```python
from build123d import *

# Parameters (mm, degrees)
SKETCH1_W           = 94
SKETCH1_H           = 130
BOSS_EXTRUDE1_DEPTH = 9.5
SKETCH2_W           = 90.5
SKETCH2_H           = 126.5
CUT_EXTRUDE1_DEPTH  = 2.5
SKETCH3_W           = 72
SKETCH3_H           = 24
CUT_EXTRUDE2_DEPTH  = 8
SKETCH4_W           = 70
SKETCH4_H           = 78
CUT_EXTRUDE3_DEPTH  = 2
SKETCH5_W           = 23
SKETCH5_H           = 3.5
CUT_EXTRUDE4_DEPTH  = 8.5
SKETCH6_W           = 6
SKETCH6_H           = 18
CUT_EXTRUDE5_DEPTH  = 3.5
SKETCH7_W           = 43
SKETCH7_H           = 7.5
CUT_EXTRUDE6_DEPTH  = 3
FILLET1_R           = 2
BOSS_EXTRUDE3_DEPTH = 2


with BuildPart() as part:
    # Sketch1 → Boss-Extrude1 (new body)
    with BuildSketch(Plane(origin=(0, 7, 0), x_dir=(1, 0, 0), z_dir=(0, 1, 0))):
        with Locations((47, 65)):
            Rectangle(SKETCH1_W, SKETCH1_H)
    extrude(amount=-BOSS_EXTRUDE1_DEPTH)

    # Sketch2 → Cut-Extrude1 (cut)
    with BuildSketch(Plane.XZ.offset(2.5)):
        with Locations((47, -65)):
            Rectangle(SKETCH2_W, SKETCH2_H)
    extrude(amount=-CUT_EXTRUDE1_DEPTH, mode=Mode.SUBTRACT)

    # Sketch3 → Cut-Extrude2 (cut, through all)
    with BuildSketch(Plane.XZ):
        with Locations((47, -100)):
            Rectangle(SKETCH3_W, SKETCH3_H)
    extrude(amount=-CUT_EXTRUDE2_DEPTH, mode=Mode.SUBTRACT)

    # Sketch4 → Cut-Extrude3 (cut)
    with BuildSketch(Plane(origin=(0, 7, 0), x_dir=(-1, 0, 0), z_dir=(0, 1, 0))):
        with Locations((-42, -44)):
            Rectangle(SKETCH4_W, SKETCH4_H)
    extrude(amount=-CUT_EXTRUDE3_DEPTH, mode=Mode.SUBTRACT)

    # Sketch5 → Cut-Extrude4 (cut, through all)
    with BuildSketch(Plane(origin=(0, 5, 0), x_dir=(-1, 0, 0), z_dir=(0, 1, 0))):
        with Locations((-42, -9.25)):
            Rectangle(SKETCH5_W, SKETCH5_H)
    extrude(amount=-CUT_EXTRUDE4_DEPTH, mode=Mode.SUBTRACT)

    # Sketch6 → Cut-Extrude5 (cut)
    with BuildSketch(Plane.XZ):
        with Locations((86, -100)):
            Rectangle(SKETCH6_W, SKETCH6_H)
    extrude(amount=-CUT_EXTRUDE5_DEPTH, mode=Mode.SUBTRACT)

    # Sketch7 → Cut-Extrude6 (cut)
    with BuildSketch(Plane.XZ):
        with Locations((33.5, -115.75)):
            Rectangle(SKETCH7_W, SKETCH7_H)
    extrude(amount=-CUT_EXTRUDE6_DEPTH, mode=Mode.SUBTRACT)

    # Fillet1
    fillet1_edges = [part.edges().sort_by_distance(p)[0] for p in [
        (94, 7, -65),
        (47, 7, 0),
        (0, 7, -65),
        (47, 7, -130),
        (94, 2.25, -130),
        (94, 2.25, 0),
        (0, 2.25, 0),
        (0, 2.25, -130),
    ]]
    fillet(fillet1_edges, radius=FILLET1_R)

    # Sketch10 → Boss-Extrude3 (add)
    with BuildSketch(Plane(origin=(0, 7, 0), x_dir=(1, 0, 0), z_dir=(0, 1, 0))):
        Polygon((26.5, 123), (24.5, 125), (20.5, 125), (18.5, 123), (18.5, 117), (20.5, 115), (24.5, 115), (25, 115.309128344), (25, 115), (26.5, 115), (26.5, 120), (22.5, 120), (22.5, 118.5), (25, 118.5), (25, 117.072659745), (24.07375083, 116.5), (21.121320344, 116.5), (20, 117.621320344), (20, 122.367836714), (21.110870681, 123.5), (23.878679656, 123.5), (25, 122.378679656), (26.5, 122.378679656), align=None)
        Polygon((32.378679656, 119), (30.5, 119), (30.5, 115), (29, 115), (29, 125), (34.5, 125), (36, 123.5), (36, 120.5), (34.5, 119), (36, 117.5), (36, 115), (34.5, 115), (34.5, 116.878679656), align=None)
        Polygon((30.5, 123.496173662), (30.5, 120.5), (33.882505994, 120.5), (34.5, 121.117494006), (34.5, 122.878679656), (33.882505994, 123.496173662), align=None, mode=Mode.SUBTRACT)
        Polygon((43.5, 125), (45.5, 123.276052985), (45.5, 117.021376869), (43.5, 115), (40.272028005, 115), (38.5, 117.021376869), (38.5, 123.276052985), (40.272028005, 125), align=None)
        Polygon((42.942743976, 123.5), (44, 122.588673317), (44, 117.638031489), (42.874003649, 116.5), (40.951839055, 116.5), (40, 117.585775983), (40, 122.642614002), (40.881298547, 123.5), align=None, mode=Mode.SUBTRACT)
        Polygon((48, 117), (50, 115), (53, 115), (55, 117), (55, 125), (53.5, 125), (53.5, 123.5), (53.5, 117.621320344), (52.378679656, 116.5), (50.621320344, 116.5), (49.5, 117.621320344), (49.5, 123.5), (49.5, 125), (48, 125), align=None)
        Polygon((63, 119), (59, 119), (59, 115), (57.5, 115), (57.5, 125), (63, 125), (64.5, 123.5), (64.5, 120.5), align=None)
        Polygon((59, 123.5), (59, 120.5), (62.378679656, 120.5), (63, 121.121320344), (63, 122.878679656), (62.378679656, 123.5), align=None, mode=Mode.SUBTRACT)
    extrude(amount=BOSS_EXTRUDE3_DEPTH)


solid = part.part
```
Can you work these out from the model? Positions are in its coordinate system, mm. A direction names the side the tool comes from. Round coordinates to 2 decimals unless told otherwise and drop trailing zeros. Loops run counter-clockwise (first coordinate to the right, second up) from the corner with the lowest first, then second, coordinate; pieces in that order, holes last.
Item 1: Suppose I cut it at C-C, the plane x = 86.5. Write out the boundary of the cut face in (y, z).
Item 2: If we mould it in two halves opening along X, with no side actions, what happens to faces 6 (the flat face through (0, 1, -64)), 7 (the flat face through (30.5, 3, -9)), 8 (the flat face through (60, 9, -120)), 9 (the flat face through (61, 7, -122))? For each: +X half, -X half, draft (parallel to the pull), parting line (faces both ways), or undercut.
Item 3: Suppose I cut it at A-A, the plane z = -102.5. Write out the boundary of the cut face in (x, y), then the cut area to 3 significant figures.
Item 4: Suppose I cut it at B-B, the plane x = 69.5. Write out the boundary of the cut face in (y, z).
Item 5: Suppose I cut it at D-D, the plane z = -66. Write out the boundary of the cut face in (x, y), then the cut area to 3 significant figures.
Item 6: Will these pins go through, and if not, where does the flat tip stop? pin 1 Ø1.6 at (x, y) = (48.5, 8) entering from -Z; pin 2 Ø0.6 at (x, y) = (51.5, 7.5) entering from +Z; pin 3 Ø2 at (x, z) = (31, -63) entering from +Y.
Item 7: Which directions (+Z, -Z, +X, -X, +Y, -Y) give clear straight access to the entire face, cutting with the end or side of a thin tool? Please do faces 1 (the flat face through (44.4, 9, -120.1)), 2 (the flat face through (94, 1, -64)), 3 (the flat face through (86, 2, -109)), 4 (the flat face through (42, 3, -7.5)), 5 (the flat face through (42, 7, -120)).
Item 8: Please list where these lines run through material, in increasing order: L1, parallel to Z at x = 11.5, y = 2; L2, parallel to Z at x = 27.5, y = 6; L3, parallel to Z at x = 55.5, y = -0.5.
Reported:
1. outline: (-2.5, -130) - (5, -130) arc R2 ccw to (7, -128) - (7, -2) arc R2 ccw to (5, 0) - (-2.5, 0) - (-2.5, -1.75) - (0, -1.75) - (0, -91) - (3.5, -91) - (3.5, -109) - (0, -109) - (0, -128.25) - (-2.5, -128.25) - close
2. face 6: -X half
2. face 7: undercut
2. face 8: draft
2. face 9: undercut
3. outline: (0, -2.5) - (1.75, -2.5) - (1.75, 0) - (11, 0) - (11, 7) - (2, 7) arc R2 ccw to (0, 5) - close; (83, 3.5) - (89, 3.5) - (89, 0) - (92.25, 0) - (92.25, -2.5) - (94, -2.5) - (94, 5) arc R2 ccw to (92, 7) - (83, 7) - close
3. area: 140 mm2
4. outline: (-2.5, -130) - (5, -130) arc R2 ccw to (7, -128) - (7, -112) - (0, -112) - (0, -128.25) - (-2.5, -128.25) - close; (-2.5, -1.75) - (0, -1.75) - (0, -88) - (7, -88) - (7, -83) - (5, -83) - (5, -5) - (7, -5) - (7, -2) arc R2 ccw to (5, 0) - (-2.5, 0) - close
5. outline: (0, -2.5) - (1.75, -2.5) - (1.75, 0) - (92.25, 0) - (92.25, -2.5) - (94, -2.5) - (94, 5) arc R2 ccw to (92, 7) - (77, 7) - (77, 5) - (7, 5) - (7, 7) - (2, 7) arc R2 ccw to (0, 5) - close
5. area: 525 mm2
6. pin 1: stops at z = -125
6. pin 2: stops at z = -115
6. pin 3: stops at y = 5
7. face 1: +Z, -Z, +X, -X, +Y
7. face 2: +Z, -Z, +X, +Y, -Y
7. face 3: -Y
7. face 4: +Y, -Y
7. face 5: +Y
8. L1: z = -130 to -112, -88 to 0
8. L2: z = -129.73 to -112, -88 to -83, -5 to -0.27
8. L3: z = -130 to -128.25, -1.75 to 0
